Geometry: final body of the model. Coordinates: model frame, mm. A direction names the side the tool comes from. Give positions to 0.01 mm unless a question says otherwise; leave off trailing zeros. Loops run counter-clockwise (first coordinate to the right, second up) from the corner with the lowest first, then second, coordinate; pieces in that order, holes last. Notation, with made-up numbers: (-32, -4.5) -> (23, -4.5) arc R35 cw to (23, 27.5) -> close; hole circle Ø8 at (79, 81). An arc over 180 degrees is marked (long way). One line per question, with ' | ' between items. Start each with the question number.
Item 1: Mould query, pull axis Y, two halves, no side actions, for faces 4 (the flat face through (0, 22, 0.8)), 5 (the cylindrical face through (0.89, 44.74, 0.39)), 6 (the cylindrical face through (-0.1, -2.7, 0.4)). Classes: released by +Y, released by -Y, zero draft, split by the parting line, or undercut.
Item 2: Section C-C on z = 0.65. Return loops of the section in (x, y) (3 decimals), then the cut area to 3 significant figures.
Item 3: Material intervals for line 1 along Y through (x, z) = (0, 0.45) (3 decimals); line 2 along Y through (x, z) = (-1.25, 0.7); line 3 along Y through (x, z) = (-1, 0.3), sorted ascending. Write a range as [from, to].
Item 4: Section B-B on x = 0.2. Return loops of the section in (y, z), then the cut area to 3 significant figures.
Item 5: Set-up query: faces 1 (the cylindrical face through (-1.732, 38.709, 0.394)), 2 (the cylindrical face through (1.715, 38.677, 0.394)), 3 (the flat face through (0, 22, 0)). Return all of +Z, -Z, +X, -X, +Y, -Y with unobstructed straight access to the full face (end or side cutting, diameter ignored); none if empty.
Item 6: Pin query (flat end, axial travel): P1, Ø1, axis at x = 0, y = 6, coming from the +Z side. Return the tip coordinate at first contact, or that it passes through.
Item 7: Section A-A on y = 6. Return loops of the section in (x, z) (3 decimals).
from build123d import *

# Parameters (mm, degrees)
SKETCH_2_R      = 1.525
SKETCH_2_R_2    = 0.825
SKETCH_2_R_3    = 1.65
EXTRUDE_1_DEPTH = 0.8


with BuildPart() as part:
    # 草图2 → 凸台-拉伸1 (new body)
    with BuildSketch(Plane.XY):
        with BuildLine():
            Line((-2.7, 33.467), (-2.7, 0))
            ThreePointArc((-2.7, 0), (0, -2.7), (2.7, 0))
            Line((2.7, 0), (2.7, 33.467))
            ThreePointArc((2.7, 33.467), (2.540401667, 33.854410039), (2.154230769, 34.016983728))
            ThreePointArc((2.154230769, 34.016983728), (1.627634091, 34.238675121), (1.41, 34.766961538))
            Line((1.41, 34.766961538), (1.41, 37.442))
            ThreePointArc((1.41, 37.442), (1.7232193, 38.69278444), (2.588946281, 39.648339169))
            ThreePointArc((2.588946281, 39.648339169), (2.670495544, 39.738349976), (2.7, 39.856170665))
            Line((2.7, 39.856170665), (2.7, 45.651))
            ThreePointArc((2.7, 45.651), (2.626776695, 45.827776695), (2.45, 45.901))
            Line((2.45, 45.901), (-2.45, 45.901))
            ThreePointArc((-2.45, 45.901), (-2.626776695, 45.827776695), (-2.7, 45.651))
            Line((-2.7, 45.651), (-2.7, 39.856170665))
            ThreePointArc((-2.7, 39.856170665), (-2.670495544, 39.738349976), (-2.588946281, 39.648339169))
            ThreePointArc((-2.588946281, 39.648339169), (-1.7232193, 38.69278444), (-1.41, 37.442))
            Line((-1.41, 37.442), (-1.41, 34.766961538))
            ThreePointArc((-1.41, 34.766961538), (-1.627634091, 34.238675121), (-2.154230769, 34.016983728))
            ThreePointArc((-2.154230769, 34.016983728), (-2.540401667, 33.854410039), (-2.7, 33.467))
        make_face()
        Circle(SKETCH_2_R, mode=Mode.SUBTRACT)
        with Locations((0, 6)):
            Circle(SKETCH_2_R_2, mode=Mode.SUBTRACT)
        with Locations((0, 43.351)):
            Circle(SKETCH_2_R_3, mode=Mode.SUBTRACT)
    extrude(amount=EXTRUDE_1_DEPTH)


solid = part.part
Result sheet:
1) face 4: zero draft | face 5: undercut | face 6: released by -Y
2) outline: (-2.7, 0) arc R2.7 ccw to (2.7, 0) -> (2.7, 33.467) arc R0.55 ccw to (2.154, 34.017) arc R0.75 cw to (1.41, 34.767) -> (1.41, 37.442) arc R2.654 cw to (2.589, 39.648) arc R0.25 ccw to (2.7, 39.856) -> (2.7, 45.651) arc R0.25 ccw to (2.45, 45.901) -> (-2.45, 45.901) arc R0.25 ccw to (-2.7, 45.651) -> (-2.7, 39.856) arc R0.25 ccw to (-2.589, 39.648) arc R2.654 cw to (-1.41, 37.442) -> (-1.41, 34.767) arc R0.75 cw to (-2.154, 34.017) arc R0.55 ccw to (-2.7, 33.467) -> close; hole circle Ø3.3 at (0, 43.351); hole circle Ø3.05 at (0, 0); hole circle Ø1.65 at (0, 6) | area: 228 mm²
3) line 1: y = [-2.7, -1.525], [1.525, 5.175], [6.825, 41.701], [45.001, 45.901] | line 2: y = [-2.39, -0.87], [0.87, 42.27], [44.43, 45.9] | line 3: y = [-2.51, -1.15], [1.15, 42.04], [44.66, 45.9]
4) outline: (-2.69, 0) -> (-1.51, 0) -> (-1.51, 0.8) -> (-2.69, 0.8) -> close; (1.51, 0) -> (5.2, 0) -> (5.2, 0.8) -> (1.51, 0.8) -> close; (6.8, 0) -> (41.71, 0) -> (41.71, 0.8) -> (6.8, 0.8) -> close; (44.99, 0) -> (45.9, 0) -> (45.9, 0.8) -> (44.99, 0.8) -> close | area: 32.6 mm²
5) face 1: +Z, -Z, -X | face 2: +Z, -Z, +X | face 3: -Z, +X, -X, +Y, -Y
6) P1: passes through
7) outline: (-2.7, 0) -> (-0.825, 0) -> (-0.825, 0.8) -> (-2.7, 0.8) -> close; (0.825, 0) -> (2.7, 0) -> (2.7, 0.8) -> (0.825, 0.8) -> close
